```python
from build123d import *
from OCP.BRepAlgoAPI import BRepAlgoAPI_Cut
from OCP.TopTools import TopTools_ListOfShape

# Parameters (mm, degrees)
BOSS_EXTRUDE2_DEPTH = 6
SKETCH3_4_R         = 8.000000000000005
SKETCH3_4_R_2       = 6.050000000000002
BOSS_EXTRUDE3_DEPTH = 3
FILLET3_R           = 3
SKETCH7_R           = 5
CUT_EXTRUDE2_DEPTH  = 10
FILLET4_START       = -11
FILLET4_DEPTH       = 22


with BuildPart() as part:
    # Sketch3 → Boss-Extrude2 (new, symmetric)
    with BuildSketch(Plane(origin=(0, 0, 0), x_dir=(1, 0, 0), z_dir=(0, 1, 0))):
        with BuildLine():
            Line((8, -10), (8, 10))
            ThreePointArc((8.000000000000002, 10), (-4.43e-15, 1.9999999999999964), (-8.000000000000009, 10.000000000000004))
            Line((-8, 10), (-8, -10))
            Line((-8, -10), (8, -10))
        make_face()
    extrude(amount=BOSS_EXTRUDE2_DEPTH, both=True)

    # Sketch3<4> → Boss-Extrude3 (add, symmetric)
    with BuildSketch(Plane(origin=(0, 0, 0), x_dir=(1, 0, 0), z_dir=(0, 1, 0))):
        with Locations((-2.96e-15, 10.000000000000002)):
            Circle(SKETCH3_4_R)
        with Locations(Location((-2.96e-15, 10.000000000000002, 0), (0, 0, 270))):
            Circle(SKETCH3_4_R_2, mode=Mode.SUBTRACT)
    extrude(amount=BOSS_EXTRUDE3_DEPTH, both=True)

    # Fillet3
    fillet3_edges = [part.edges().sort_by_distance(p)[0] for p in [
        (-5.06e-15, -6, -1.9999999999999947),
        (-5.06e-15, 6, -1.9999999999999947),
    ]]
    fillet(fillet3_edges, radius=FILLET3_R - 0.0001)  # a hair under: the kernel refuses the full size

    # Sketch7 → Cut-Extrude2 (cut)
    with BuildSketch(Plane.XY.offset(10)):
        Circle(SKETCH7_R)
    extrude(amount=-CUT_EXTRUDE2_DEPTH, mode=Mode.SUBTRACT)


with BuildPart() as fillet4_tool:
    # Fillet4: read off the stored shape, not the designer's step
    # Fillet4 outline → Fillet4 (new body)
    with BuildSketch(Plane.XY.offset(FILLET4_START)):
        with BuildLine():
            Line((-8, 6), (-8, 3))
            ThreePointArc((-8, 3), (-7.121320344, 5.121320344), (-5, 6))
            Line((-5, 6), (-8, 6))
        make_face()
        with BuildLine():
            ThreePointArc((-5, -6), (-7.121320344, -5.121320344), (-8, -3))
            Line((-8, -3), (-8, -6))
            Line((-8, -6), (-5, -6))
        make_face()
        with BuildLine():
            Line((8, 6), (5, 6))
            ThreePointArc((5, 6), (7.121320344, 5.121320344), (8, 3))
            Line((8, 3), (8, 6))
        make_face()
        with BuildLine():
            ThreePointArc((8, -3), (7.121320344, -5.121320344), (5, -6))
            Line((5, -6), (8, -6))
            Line((8, -6), (8, -3))
        make_face()
    extrude(amount=FILLET4_DEPTH)


with BuildPart() as part_1:
    add(part.part)

    # Fillet4: cut by fillet4_tool, with a tolerance
    fillet4_stock = TopTools_ListOfShape()
    fillet4_stock.Append(part_1.part.wrapped)
    fillet4_tools = TopTools_ListOfShape()
    fillet4_tools.Append(fillet4_tool.part.wrapped)
    fillet4_cut = BRepAlgoAPI_Cut()
    fillet4_cut.SetArguments(fillet4_stock)
    fillet4_cut.SetTools(fillet4_tools)
    fillet4_cut.SetFuzzyValue(0.00001)
    fillet4_cut.Build()
    add(Compound.cast(fillet4_cut.Shape()).solids(), mode=Mode.REPLACE)


solid = part_1.part
```
The listing builds one solid part. Answer for the finished solid, in the listing's coordinates (mm). A direction names the side the tool comes from. Round coordinates to 2 decimals unless told otherwise and drop trailing zeros. Loops run counter-clockwise (first coordinate to the right, second up) from the corner with the lowest first, then second, coordinate; pieces in that order, holes last.
1) For faces 4 (the face through (-2, 3, -16)), 5 (the face through (-2, -3, -16)), 6 (the face through (0, 0, 0)), 7 (the face through (0, -6, 5)), determine the directions among +Z, -Z, +X, -X, +Y, -Y from which every point of the face is accessible in a straight line to the end or side of a thin tool.
Outcome:
face 4: -Z, +Y
face 5: -Z, -Y
face 6: +Z
face 7: +Z, -Z, +X, -X, -Y
2) A cutting plane is placed at C-C on y = 1.5. Determine the outline of the cut face in (x, z).
Outcome:
outline: (-8, -10) arc R8 ccw to (8, -10) - (8, 10) - (4.77, 10) - (4.77, 0) - (-4.77, 0) - (-4.77, 10) - (-8, 10) - close; hole circle Ø12.1 at (0, -10)
3) A cutting plane is placed at B-B on z = 6.5. Determine the outline of the cut face in (x, y), plus the area to 3 significant figures.
Outcome:
outline: (-8, -3) arc R3 ccw to (-5, -6) - (5, -6) arc R3 ccw to (8, -3) - (8, 3) arc R3 ccw to (5, 6) - (-5, 6) arc R3 ccw to (-8, 3) - close; hole circle Ø10 at (0, 0)
area: 106 mm2
4) For a pull along Z with two mould halves and no side action, classify faces 1 (the face through (-3.68, -0.04, -14.8)), 2 (the face through (7.48, -4.69, 2.08)), 3 (the face through (0, 0, -18)) as released by +Z, released by -Z, zero draft, split by the parting line, or undercut.
Outcome:
face 1: undercut
face 2: zero draft
face 3: released by -Z
5) Given P1, Ø2, axis at x = -4.5, y = 0, coming from the -Z side; P2, Ø3, axis at x = -0.5, y = 2.5, coming from the +Z side; P3, Ø5, axis at x = 2.5, z = -10.5, coming from the -Y side; P4, Ø8, axis at x = -2.5, z = -11.5, coming from the +Y side, each flat-ended and moving along its own axis, determine where each tip first touches the part or whether it passes through.
Outcome:
P1: stops at z = -17.19
P2: stops at z = 0
P3: passes through
P4: stops at y = 3
6) Consider line 1 (X direction, y = 1.6, z = -10); line 2 (Y direction, x = 0, z = 5); line 3 (Y direction, x = -4.25, z = -4.75). Determine where each line is inside the solid, lowest interval first.
Outcome:
line 1: x = -8 to -6.05, 6.05 to 8
line 2: y = -6 to -5, 5 to 6
line 3: y = -3 to 3
7) A cutting plane is placed at A-A on x = 0. Determine the outline of the cut face in (y, z).
Outcome:
outline: (-6, 1) arc R3 ccw to (-3, -2) - (-3, -3.95) - (3, -3.95) - (3, -2) arc R3 ccw to (6, 1) - (6, 10) - (5, 10) - (5, 0) - (-5, 0) - (-5, 10) - (-6, 10) - close; (-3, -18) - (3, -18) - (3, -16.05) - (-3, -16.05) - close
